Autodesk Inventor part; units mm, degrees
ref_plane "YZ Plane" through (0, 0, 0) normal (1, 0, 0) x (0, 1, 0)
ref_plane "XZ Plane" through (0, 0, 0) normal (0, 1, 0) x (-1, 0, 0)
ref_plane "XY Plane" through (0, 0, 0) normal (0, 0, 1) x (1, 0, 0)
sketch "Sketch3" plane through (0, 0, 0) normal (0, 0, 1) x (1, 0, 0)
  line L0 (0, 0) -> (27.5, 0)
  line L1 (27.5, 0) -> (27.5, 15)
  line L2 (0, 32.6777) -> (0, 0)
  line L3 (0, 39) -> (0, 109)
  line L4 (5, 109) -> (9.8223, 109)
  line L5 (9.8223, 109) -> (9.8223, 39)
  line L6 (0, 109) -> (5, 109) construction
  line L7 (5, 109) -> (5, 114)
  line L8 (5, 114) -> (0, 114)
  line L9 (0, 114) -> (0, 109)
  line L10 (27.5, 15) -> (9.8223, 39)
  line L11 (0, 32.6777) -> (0, 39)
  dimension "d5" = 27.5
  dimension "d6" = 15
  dimension "d10" = 70
  dimension "d14" = 5
  dimension "d15" = 5
revolve "Revolution1" add sketch "Sketch3" angle 360 about axis through (0, 32.6777, 0) along (0, -1, 0)
sketch "Sketch5" plane through (0, 114, 0) normal (0, 1, 0) x (1, 0, 0)
  line L0 (0, 0) -> (0, 8) construction
  line L1 (0, 8) -> (-8, 8)
  line L2 (-8, 8) -> (-8, -37)
  line L3 (-8, -37) -> (8, -37)
  line L4 (8, -37) -> (8, 8)
  line L5 (8, 8) -> (0, 8)
  dimension "d16" = 8
  dimension "d17" = 8
  dimension "d18" = 45
  dimension "d19" = 16
extrude "Extrusion1" add sketch "Sketch5" along normal blind 31
sketch "Sketch6" plane through (8, 114, 37) normal (1, 0, 0) x (0, 0, -1)
  line L0 (0, 31) -> (11, 31) construction
  line L1 (0, 31) -> (45, 31) construction
  line L2 (11, 31) -> (11, 27) construction
  line L3 (11, 31) -> (31, 31) construction
  line L4 (31, 31) -> (31, 27) construction
  circle A0 centre (11, 27) radius 2.75
  circle A1 centre (31, 27) radius 2.75
  point P0 (37, -114)
  point P1 (22.5, 31)
  point P2 (0, 31)
  dimension "d28" = 11
  dimension "d29" = 20
extrude "Extrusion2" cut sketch "Sketch6" against normal blind 16
properties part number "Suction"
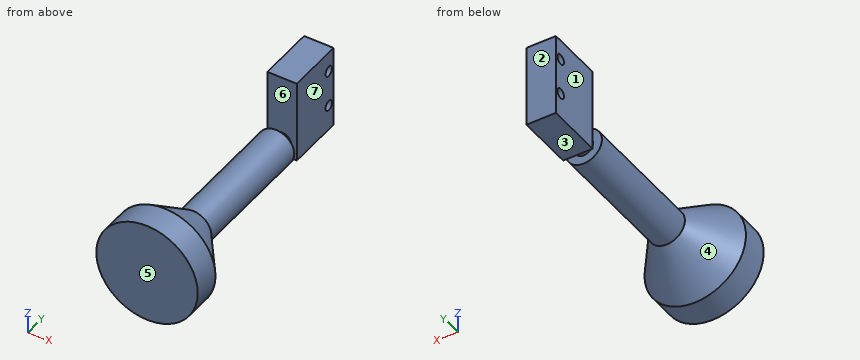
Verification items for the finished model (mm, model axes). Face numbers are marked on the shaded views. A direction names the side the tool comes from. Coordinates: 2 decimals unless noted, no trailing zeros. Loops run counter-clockwise (first coordinate to the right, second up) from the corner with the lowest first, then second, coordinate; pieces in that order, holes last. Notation, with made-up numbers: (35, 47) - (86, 47) arc R19 ccw to (86, 55) - close; hole circle Ø8 at (63.5, 62.25). An arc over 180 degrees is marked (long way). Return JSON: item names as keys, results as strings.
1. Section check D-D, the plane y = 123. Record the boundary of the cut face in (x, z), then the cut area to 3 significant figures.
Established:
{"outline": "(-8, -8) - (8, -8) - (8, 37) - (-8, 37) - close", "area": "720 mm2"}
2. Go/stop test with flat-tipped pins: pin 1 (2 mm diameter, centred on y = 16.5, z = -3.5, fed in from +X); pin 2 (15.5 mm diameter, centred on y = 130.5, z = 16, fed in from +X); pin 3 (8 mm diameter, centred on x = 3, y = 136, fed in from -Z). Record where each tip stops, or that it passes through.
Established:
{"pin 1": "stops at x = 26.92", "pin 2": "stops at x = 8", "pin 3": "stops at z = -8"}
3. Section check A-A, the plane y = 141. Record the boundary of the cut face in (x, z).
Established:
{"outline": "(-8, -8) - (8, -8) - (8, 3.25) - (-8, 3.25) - close; (-8, 8.75) - (8, 8.75) - (8, 23.25) - (-8, 23.25) - close; (-8, 28.75) - (8, 28.75) - (8, 37) - (-8, 37) - close"}
4. Section check C-C, the plane z = 31. Record the boundary of the cut face in (x, y), then the cut area to 3 significant figures.
Established:
{"outline": "(-8, 114) - (8, 114) - (8, 145) - (-8, 145) - close", "area": "496 mm2"}
5. Mould release check, pull along Y, two halves, no side actions. Record for the marked faces 5, 6 and 7: +Y half, -Y half, draft (parallel to the pull), parting line (faces both ways), or undercut.
Established:
{"face 5": "-Y half", "face 6": "undercut", "face 7": "draft"}
6. Tool access check on the marked faces 1, 2, 3 and 4. Record the directions out of +Z, -Z, +X, -X, +Y, -Y that give a thin tool (end or side, any length) a straight path to the whole face; none if there is none.
Established:
{"face 1": "+Z, -Z, -X, +Y", "face 2": "+Z, -Z, +X, -X, +Y", "face 3": "-Z, +X, -X, +Y", "face 4": "none"}
7. Section check B-B, the plane x = 0. Record the boundary of the cut face in (y, z), then the cut area to 3 significant figures.
Established:
{"outline": "(0, -27.5) - (15, -27.5) - (39, -9.82) - (109, -9.82) - (109, -5) - (114, -5) - (114, -8) - (145, -8) - (145, 37) - (114, 37) - (114, 5) - (109, 5) - (109, 9.82) - (39, 9.82) - (15, 27.5) - (0, 27.5) - close; hole circle Ø5.5 at (141, 6); hole circle Ø5.5 at (141, 26)", "area": "4,490 mm2"}
8. Thickness scan on L1, parallel to Z at x = 4, y = 141; L2, parallel to Y at x = -1, z = 26; L3, parallel to Y at x = -2, z = 6. Record the ranges inside material, lowest first.
Established:
{"L1": "z = -8 to 3.25, 8.75 to 23.25, 28.75 to 37", "L2": "y = 0 to 17.01, 114 to 138.25, 143.75 to 145", "L3": "y = 0 to 109, 114 to 138.25, 143.75 to 145"}
